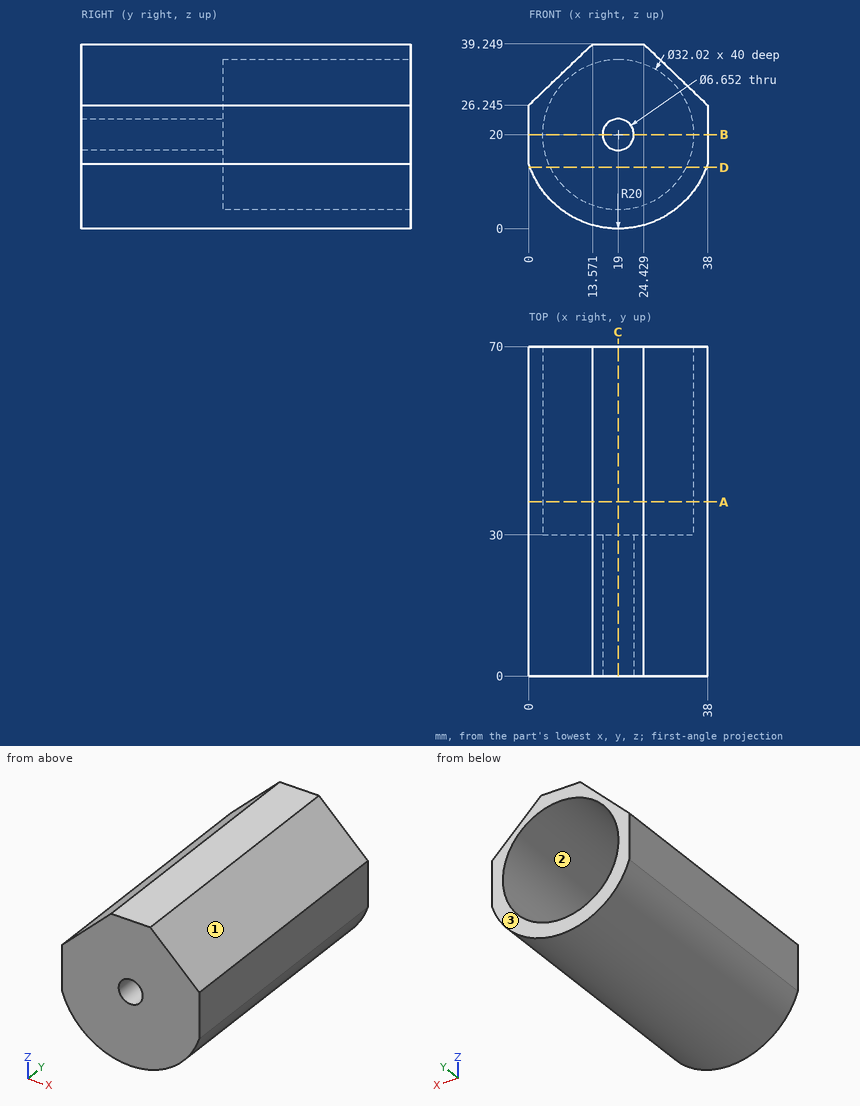
Part print with two shaded views. Sizes in mm from the minimum x, y, z corner. Give positions to 0.01 mm unless a question says otherwise; leave off trailing zeros. Loops run counter-clockwise (first coordinate to the right, second up) from the corner with the lowest first, then second, coordinate; pieces in that order, holes last. Notation, with made-up numbers: (24.5, 64.25) - (79.5, 64.25) arc R28 ccw to (79.5, 84.25) - close; hole circle Ø3 at (-14.75, 78.25). An arc over 180 degrees is marked (long way). Put each result on its own line as item: value.
Q1. Flat gauge pins, fed straight in: pin 1 (12 mm diameter, centred on x = 16.5, z = 19, fed in from +Y); pin 2 (8 mm diameter, centred on y = 38, z = 5.5, fed in from -X); pin 3 (1 mm diameter, centred on x = 18, y = 31.5, fed in from -Z). Where does each tip first touch, or does it go through?
Filled in:
pin 1: stops at y = 30
pin 2: stops at x = 1.98
pin 3: stops at z = 0.01
Q2. Probe line 1 along X through (y, z) = (9, 20); line 2 along Y through (x, z) = (14, 18); line 3 along X through (y, z) = (45, 20). List the from-to ranges inside material, lowest first.
Filled in:
line 1: x = 0 to 15.67, 22.33 to 38
line 2: y = 0 to 30
line 3: x = 0 to 2.99, 35.01 to 38
Q3. Slice it at A-A (y = 37). Give the cut face in (x, z) (1 decimal).
Filled in:
outline: (0, 13.8) arc R20 ccw to (38, 13.8) - (38, 26.2) - (24.4, 39.2) - (13.6, 39.2) - (0, 26.2) - close; hole circle Ø32 at (19, 20)
Q4. Slice it at D-D (z = 13). Give the cut face in (x, y) (1 decimal).
Filled in:
outline: (0.3, 0) - (37.7, 0) - (37.7, 70) - (33.4, 70) - (33.4, 30) - (4.6, 30) - (4.6, 70) - (0.3, 70) - close
Q5. Slice it at C-C (x = 19). Give the cut face in (y, z).
Filled in:
outline: (0, 0) - (70, 0) - (70, 3.99) - (30, 3.99) - (30, 16.67) - (0, 16.67) - close; (0, 23.33) - (30, 23.33) - (30, 36.01) - (70, 36.01) - (70, 39.25) - (0, 39.25) - close
Q6. Mould opens along Z. For the marked faces 1, 2 and 3 say: pulls with the +Z half, pulls with the -Z half, needs draft (parallel to the pull), parting line crosses it, or undercut.
Filled in:
face 1: pulls with the +Z half
face 2: undercut
face 3: needs draft
Q7. Slice it at B-B (z = 20). Give the cut face in (x, y).
Filled in:
outline: (0, 0) - (15.67, 0) - (15.67, 30) - (2.99, 30) - (2.99, 70) - (0, 70) - close; (22.33, 0) - (38, 0) - (38, 70) - (35.01, 70) - (35.01, 30) - (22.33, 30) - close
